Geometry: final body of the model. Coordinates: model frame, mm. Give positions to 0.01 mm unless a question says otherwise; leave off trailing zeros. Order: outer loops, then holes, each group sorted by start corner. A loop starts at its lowest first (then second) coordinate and runs counter-clockwise, first axis right, second up. Notation, with made-up numbers: (40, -24.5) -> (81, -24.5) arc R19 cw to (81, -4.5) -> close; hole circle Ø9 at (69.25, -23). An arc over 180 degrees is marked (long way). One line per question, with ' | ' between items.
from build123d import *

# Parameters (mm, degrees)
ESBO_O1_W                = 175
ESBO_O1_H                = 172.5
RESSALTO_EXTRUS_O1_DEPTH = 10
ESBO_O5_W                = 30
ESBO_O5_H                = 6
RESSALTO_EXTRUS_O5_DEPTH = 10
ESBO_O6_W                = 6
ESBO_O6_H                = 30
RESSALTO_EXTRUS_O6_DEPTH = 10
ESBO_O7_W                = 30
ESBO_O7_H                = 6
RESSALTO_EXTRUS_O7_DEPTH = 10
ESBO_O8_W                = 6.3
ESBO_O8_H                = 172.5
CORTE_EXTRUS_O1_DEPTH    = 5
ESBO_O9_R                = 1.5
CORTE_EXTRUS_O2_DEPTH    = 8
ESBO_O10_R               = 1.5
CORTE_EXTRUS_O3_DEPTH    = 8
CORTE_EXTRUS_O4_DEPTH    = 11


with BuildPart() as part:
    # Esboço1 → Ressalto-extrusão1 (new body)
    with BuildSketch(Plane.XY):
        Rectangle(ESBO_O1_W, ESBO_O1_H)
    extrude(amount=RESSALTO_EXTRUS_O1_DEPTH)

    # Esboço5 → Ressalto-extrusão5 (add)
    with BuildSketch(Plane(origin=(0, 86.25, 0), x_dir=(1, 0, 0), z_dir=(0, 1, 0))):
        with Locations((-37.5, -5)):
            Rectangle(ESBO_O5_W, ESBO_O5_H)
        with Locations((37.5, -5)):
            Rectangle(ESBO_O5_W, ESBO_O5_H)
    extrude(amount=RESSALTO_EXTRUS_O5_DEPTH)

    # Esboço6 → Ressalto-extrusão6 (add)
    with BuildSketch(Plane.ZY.offset(87.5)):
        with Locations((5, 36.25)):
            Rectangle(ESBO_O6_W, ESBO_O6_H)
        with Locations((5, -36.25)):
            Rectangle(ESBO_O6_W, ESBO_O6_H)
    extrude(amount=RESSALTO_EXTRUS_O6_DEPTH)

    # Esboço7 → Ressalto-extrusão7 (add)
    with BuildSketch(Plane.XZ.offset(86.25)):
        with Locations((-37.5, 5)):
            Rectangle(ESBO_O7_W, ESBO_O7_H)
        with Locations((37.5, 5)):
            Rectangle(ESBO_O7_W, ESBO_O7_H)
    extrude(amount=RESSALTO_EXTRUS_O7_DEPTH)

    # Esboço8 → Corte-extrusão1 (cut)
    with BuildSketch(Plane(origin=(0, 0, 0), x_dir=(-1, 0, 0), z_dir=(0, 0, -1))):
        with Locations((-79.35, 0)):
            Rectangle(ESBO_O8_W, ESBO_O8_H)
    extrude(amount=-CORTE_EXTRUS_O1_DEPTH, mode=Mode.SUBTRACT)

    # Esboço9 → Corte-extrusão2 (cut)
    with BuildSketch(Plane.ZY.offset(87.5)):
        with Locations((5, -71.25)):
            Circle(ESBO_O9_R)
    extrude(amount=-CORTE_EXTRUS_O2_DEPTH, mode=Mode.SUBTRACT)

    # Esboço10 → Corte-extrusão3 (cut)
    with BuildSketch(Plane.XZ.offset(86.25)):
        with Locations((65, 5)):
            Circle(ESBO_O10_R)
    extrude(amount=-CORTE_EXTRUS_O3_DEPTH, mode=Mode.SUBTRACT)

    # Esboço11 → Corte-extrusão4 (cut, through all)
    with BuildSketch(Plane.XY.offset(10)):
        with BuildLine():
            ThreePointArc((3.85, 7.31931366), (-5.25, 3.75), (3.85, 0.18068634))
            Line((3.85, 0.18068634), (3.85, 7.31931366))
        make_face()
    extrude(amount=-CORTE_EXTRUS_O4_DEPTH, mode=Mode.SUBTRACT)


solid = part.part
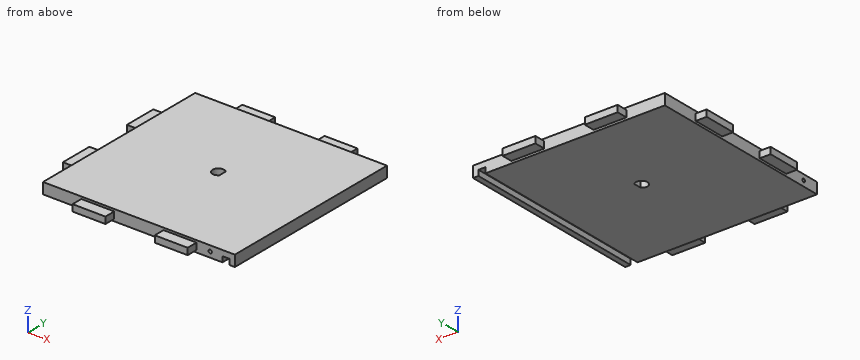
1) Section A-A on y = 3.75. Return loops of the section in (x, z).
Check result:
outline: (-87.5, 0) -> (-5.25, 0) -> (-5.25, 10) -> (-87.5, 10) -> close; (3.85, 0) -> (76.2, 0) -> (76.2, 5) -> (82.5, 5) -> (82.5, 0) -> (87.5, 0) -> (87.5, 10) -> (3.85, 10) -> close
2) Contact query for flat-ended pins moving along their axis: pin 1 Ø5 at (y, z) = (93.5, 3.5) entering from +X; pin 2 Ø3.5 at (y, z) = (5.5, 4) entering from -X; pin 3 Ø1.5 at (y, z) = (-71.5, 5) entering from -X. Output: stop coordinate, or through.
Check result:
pin 1: stops at x = 52.5 | pin 2: stops at x = -87.5 | pin 3: stops at x = -79.5
3) Material intervals for probe 1 along Y at (x, z) = (-84.25, 5); probe 2 along X at (y, z) = (4, 7); probe 3 along X at (y, z) = (84, 4), sorted ascending. Write a range as from..to.
Check result:
probe 1: y = -86.25..-72.75, -69.75..86.25 | probe 2: x = -87.5..-5.24, 3.85..87.5 | probe 3: x = -87.5..76.2, 82.5..87.5
4) Section C-C on x = 29.5. Return loops of the section in (y, z), plus the area to 4 significant figures.
Check result:
outline: (-96.25, 2) -> (-86.25, 2) -> (-86.25, 0) -> (86.25, 0) -> (86.25, 2) -> (96.25, 2) -> (96.25, 8) -> (86.25, 8) -> (86.25, 10) -> (-86.25, 10) -> (-86.25, 8) -> (-96.25, 8) -> close | area: 1,845 mm^2
5) Section D-D on x = 60. Return loops of the section in (y, z), plus the area to 4 significant figures.
Check result:
outline: (-86.25, 0) -> (86.25, 0) -> (86.25, 10) -> (-86.25, 10) -> close | area: 1,725 mm^2
6) Section B-B on y = -26. Return loops of the section in (x, z).
Check result:
outline: (-97.5, 2) -> (-87.5, 2) -> (-87.5, 0) -> (76.2, 0) -> (76.2, 5) -> (82.5, 5) -> (82.5, 0) -> (87.5, 0) -> (87.5, 10) -> (-87.5, 10) -> (-87.5, 8) -> (-97.5, 8) -> close
